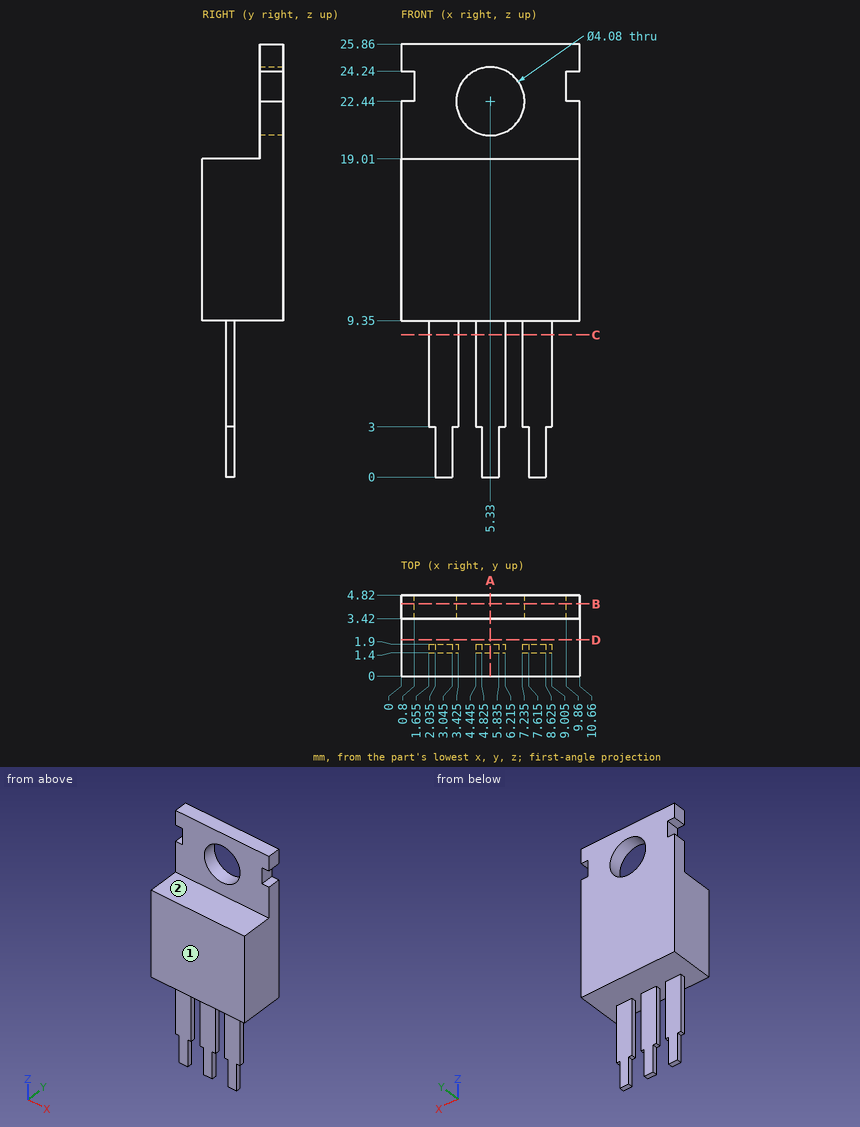
Input: dimensioned drawing with shaded views. Units: mm. Origin: part minimum x, y, z. A direction names the side the tool comes from. Round coordinates to 2 decimals unless told otherwise and drop trailing zeros. Loops run counter-clockwise (first coordinate to the right, second up) from the corner with the lowest first, then second, coordinate; pieces in that order, holes last. Notation, with made-up numbers: (30, 26) -> (48, 26) arc R17 cw to (48, 31) -> close; hole circle Ø1 at (4, 80). An arc over 180 degrees is marked (long way). Answer as a JSON object with one key per item and string values. Group by question number.
1) Section query C-C on z = 8.5. Output: boundary loops of the cut face in (x, y) (3 decimals), plus the area to 4 significant figures.
2) Section query B-B on y = 4.3. Output: boundary loops of the cut face in (x, z), plus the area to 3 significant figures.
3) Reachability of the marked faces 1 and 2 from +Z, -Z, +X, -X, +Y, -Y: full face, straight path, thin tool, end or side. Return the list, or none.
4) Section query A-A on x = 5.33. Output: boundary loops of the cut face in (y, z), plus the area to 3 significant figures.
5) Section query D-D on y = 2.15. Output: boundary loops of the cut face in (x, z).
6) Ray query, L1, parallel to Z at x = 5.33, y = 4; L2, parallel to Z at x = 8.5, y = 2.7; L3, parallel to Z at x = 2.5, y = 3.8. Return the intervals inside material, ascending.
7) Pin query (flat end, axial travel): pin 1 (0.9 mm diameter, centred on x = 2.5, z = 5.5, fed in from +Y); pin 2 (2.5 mm diameter, centred on x = 5.33, z = 22.44, fed in from +Y); pin 3 (1.5 mm diameter, centred on x = 8.5, y = 4, fed in from -Z); pin 4 (0.6 mm diameter, centred on y = 2, z = 1, fed in from +X) (3 decimals). Return the tip coordinate at first contact, or that it passes through.
Reply:
{
 "1": {"outline": "(1.655, 1.4) -> (3.425, 1.4) -> (3.425, 1.9) -> (1.655, 1.9) -> close; (4.445, 1.4) -> (6.215, 1.4) -> (6.215, 1.9) -> (4.445, 1.9) -> close; (7.235, 1.4) -> (9.005, 1.4) -> (9.005, 1.9) -> (7.235, 1.9) -> close", "area": "2.655 mm2"},
 "2": {"outline": "(0, 9.35) -> (10.66, 9.35) -> (10.66, 22.44) -> (9.86, 22.44) -> (9.86, 24.24) -> (10.66, 24.24) -> (10.66, 25.86) -> (0, 25.86) -> (0, 24.24) -> (0.8, 24.24) -> (0.8, 22.44) -> (0, 22.44) -> close; hole circle Ø4.08 at (5.33, 22.44)", "area": "160 mm2"},
 "3": {"face 1": "+Z, -Z, +X, -X, -Y", "face 2": "+Z, +X, -X, -Y"},
 "4": {"outline": "(0, 9.35) -> (1.4, 9.35) -> (1.4, 0) -> (1.9, 0) -> (1.9, 9.35) -> (4.82, 9.35) -> (4.82, 20.4) -> (3.42, 20.4) -> (3.42, 19.01) -> (0, 19.01) -> close; (3.42, 24.48) -> (4.82, 24.48) -> (4.82, 25.86) -> (3.42, 25.86) -> close", "area": "55.1 mm2"},
 "5": {"outline": "(0, 9.35) -> (10.66, 9.35) -> (10.66, 19.01) -> (0, 19.01) -> close"},
 "6": {"L1": "z = 9.35 to 20.4, 24.48 to 25.86", "L2": "z = 9.35 to 19.01", "L3": "z = 9.35 to 25.86"},
 "7": {"pin 1": "stops at y = 1.9", "pin 2": "passes through", "pin 3": "stops at z = 9.35", "pin 4": "stops at x = 8.625"}
}
